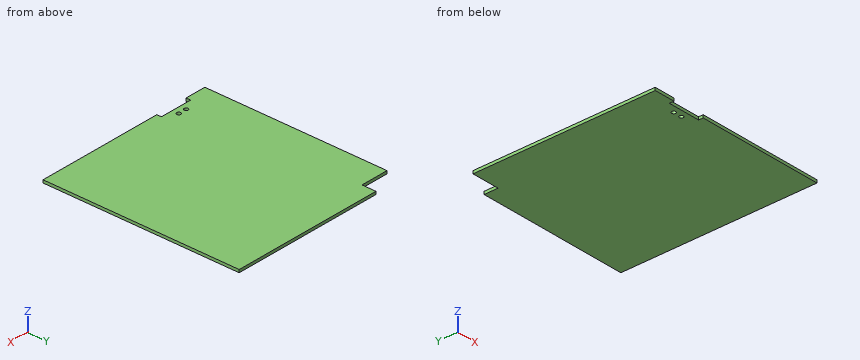
```python
from build123d import *

# Parameters (mm, degrees)
SKETCH_1_W               = 180
SKETCH_1_H               = 195
EXTRUDE_1_DEPTH          = 3
CUT_EXTRUDE_1_DEPTH      = 133.722454769
CUT_EXTRUDE_1_DEPTH_BACK = 133.722454769
SKETCH_2_R               = 2.15
SKETCH_3_W               = 10
SKETCH_3_H               = 195
EXTRUDE_2_DEPTH          = 3
SKETCH_4_W               = 116
SKETCH_4_H               = 22
EXTRUDE_3_DEPTH          = 3
CUT_EXTRUDE_2_DEPTH      = 156.850088226
CUT_EXTRUDE_2_DEPTH_BACK = 156.850088226
SKETCH_5_W               = 116
SKETCH_5_H               = 7
CUT_EXTRUDE_3_DEPTH      = 151.549825639
CUT_EXTRUDE_3_DEPTH_BACK = 151.549825639
CUT_EXTRUDE_4_DEPTH      = 150.06122903
CUT_EXTRUDE_4_DEPTH_BACK = 150.06122903
SKETCH_7_W               = 188
SKETCH_7_H               = 38.626728851
EXTRUDE_4_DEPTH          = 3
CUT_EXTRUDE_5_DEPTH      = 159.937880947
CUT_EXTRUDE_5_DEPTH_BACK = 159.937880947
SKETCH_9_W               = 6
SKETCH_9_H               = 195.373271149
SKETCH_11_W              = 164
SKETCH_11_H              = 15
EXTRUDE_5_DEPTH          = 3


with BuildPart() as part:
    # 草图1 → 凸台-拉伸1 (new body)
    with BuildSketch(Plane.XY):
        Rectangle(SKETCH_1_W, SKETCH_1_H)
    extrude(amount=EXTRUDE_1_DEPTH)

    # 草图2 → 切除-拉伸1 (cut, two sides: drawn at the far end of the back side and taken through both)
    with BuildSketch(Plane.XY.offset(3).offset(-CUT_EXTRUDE_1_DEPTH_BACK)):
        with Locations((-58.5, -60.1)):
            Circle(SKETCH_2_R)
        with Locations((-49.5, -60.1)):
            Circle(SKETCH_2_R)
        Polygon((-71.5, -67), (-67.7, -67), (-40.3, -67), (-36.5, -67), (-36.5, -72.5), (-26, -72.5), (-26, -97.5), (-82, -97.5), (-82, -72.5), (-71.5, -72.5), align=None)
    extrude(amount=CUT_EXTRUDE_1_DEPTH + CUT_EXTRUDE_1_DEPTH_BACK, mode=Mode.SUBTRACT)

    # 草图3 → 凸台-拉伸2 (add)
    with BuildSketch(Plane.XY.offset(3)):
        with Locations((-95, 0)):
            Rectangle(SKETCH_3_W, SKETCH_3_H)
    extrude(amount=-EXTRUDE_2_DEPTH)

    # 草图4 → 凸台-拉伸3 (add)
    with BuildSketch(Plane(origin=(0, 0, 0), x_dir=(-1, 0, 0), z_dir=(0, 0, -1))):
        with Locations((-32, -108.5)):
            Rectangle(SKETCH_4_W, SKETCH_4_H)
    extrude(amount=-EXTRUDE_3_DEPTH)

    # 草图5 → 切除-拉伸2 (cut, two sides: drawn at the far end of the back side and taken through both)
    with BuildSketch(Plane(origin=(0, 0, 0), x_dir=(-1, 0, 0), z_dir=(0, 0, -1)).offset(-CUT_EXTRUDE_2_DEPTH_BACK)):
        with Locations((-32, -116)):
            Rectangle(SKETCH_5_W, SKETCH_5_H)
    extrude(amount=CUT_EXTRUDE_2_DEPTH + CUT_EXTRUDE_2_DEPTH_BACK, mode=Mode.SUBTRACT)

    # 草图6 → 切除-拉伸3 (cut, two sides: drawn at the far end of the back side and taken through both)
    with BuildSketch(Plane(origin=(0, 0, 0), x_dir=(-1, 0, 0), z_dir=(0, 0, -1)).offset(-CUT_EXTRUDE_3_DEPTH_BACK)):
        Polygon((100, -97.5), (100, -95.5), (84, -95.5), (84, -72.5), (82, -72.5), (82, -97.5), align=None)
        Polygon((24, -72.5), (24, -110.5), (-88, -110.5), (-88, 95.5), (100, 95.5), (100, 97.5), (-90, 97.5), (-90, -112.5), (26, -112.5), (26, -72.5), align=None)
    extrude(amount=CUT_EXTRUDE_3_DEPTH + CUT_EXTRUDE_3_DEPTH_BACK, mode=Mode.SUBTRACT)

    # 草图7 → 切除-拉伸4 (cut, two sides: drawn at the far end of the back side and taken through both)
    with BuildSketch(Plane(origin=(0, 0, 0), x_dir=(-1, 0, 0), z_dir=(0, 0, -1)).offset(-CUT_EXTRUDE_4_DEPTH_BACK)):
        with Locations((6, -91.186635575)):
            Rectangle(SKETCH_7_W, SKETCH_7_H)
    extrude(amount=CUT_EXTRUDE_4_DEPTH + CUT_EXTRUDE_4_DEPTH_BACK, mode=Mode.SUBTRACT)

    # 草图8 → 凸台-拉伸4 (add)
    with BuildSketch(Plane(origin=(0, 0, 0), x_dir=(-1, 0, 0), z_dir=(0, 0, -1))):
        Polygon((-88, 95.5), (100, 95.5), (100, 123.5), (-80, 123.5), (-100, 123.5), (-100, -71.873271149), (-88, -71.873271149), align=None)
    extrude(amount=-EXTRUDE_4_DEPTH)

    # 草图9 → 切除-拉伸5 (cut, two sides: drawn at the far end of the back side and taken through both)
    with BuildSketch(Plane(origin=(0, 0, 0), x_dir=(-1, 0, 0), z_dir=(0, 0, -1)).offset(-CUT_EXTRUDE_5_DEPTH_BACK)):
        with Locations((97, 25.813364426)):
            Rectangle(SKETCH_9_W, SKETCH_9_H)
    extrude(amount=CUT_EXTRUDE_5_DEPTH + CUT_EXTRUDE_5_DEPTH_BACK, mode=Mode.SUBTRACT)

    # 草图11 → 凸台-拉伸5 (add)
    with BuildSketch(Plane(origin=(0, 0, 0), x_dir=(-1, 0, 0), z_dir=(0, 0, -1))):
        with Locations((-18, 131)):
            Rectangle(SKETCH_11_W, SKETCH_11_H)
    extrude(amount=-EXTRUDE_5_DEPTH)


solid = part.part
```
Work out the finished part from the listing and answer in its coordinate system (mm). Give positions to 0.01 mm unless a question says otherwise; leave off trailing zeros. Loops run counter-clockwise (first coordinate to the right, second up) from the corner with the lowest first, then second, coordinate; pieces in that order, holes last. Notation, with made-up numbers: (-9.5, 4) -> (48.5, 4) arc R14 cw to (48.5, 31) -> close; hole circle Ø6 at (-27.5, -5). An arc over 180 degrees is marked (long way). Use CSV: the item, a comma, the result in double quotes.
1. Straight lines are drawn through the part: line 1 (X direction, y = -60.1, z = 1.5); line 2 (Y direction, x = -58.5, z = 1.85); line 3 (Y direction, x = -83.5, z = 2.55). For each, find the intervals that lie inside material, in ascending order.
Found:
line 1,"-94 to -60.65, -56.35 to -51.65, -47.35 to 100"
line 2,"-67 to -62.25, -57.95 to 138.5"
line 3,"-71.87 to 123.5"
2. Flat-ended cylindrical pins translate along their axes: pin 1 Ø3.5 at (x, y) = (-49.5, -60.1) entering from -Z; pin 2 Ø0.9 at (x, z) = (-80.5, 1) entering from +Y. Find the tip coordinate at first contact, or state that the pin passes through.
Found:
pin 1,"through"
pin 2,"y = 123.5"
3. The part is cut by section A-A (z = 1.45). Write down the section's boundary in (x, y).
Found:
outline,"(-94, -71.87) -> (-71.5, -71.87) -> (-71.5, -67) -> (-36.5, -67) -> (-36.5, -71.87) -> (100, -71.87) -> (100, 138.5) -> (-64, 138.5) -> (-64, 123.5) -> (-94, 123.5) -> close; hole circle Ø4.3 at (-58.5, -60.1); hole circle Ø4.3 at (-49.5, -60.1)"
4. The part is cut by section B-B (x = -79.5). Write down the section's boundary in (y, z).
Found:
outline,"(-71.87, 0) -> (123.5, 0) -> (123.5, 3) -> (-71.87, 3) -> close"
